from build123d import *

# Parameters (mm, degrees)
FILLET_1_R = 1


with BuildPart() as part:
    # Эскиз2 → Повернуть1 (revolve)
    with BuildSketch(Plane(origin=(0, 0, 0), x_dir=(0, 0, -1), z_dir=(1, 0, 0)), mode=Mode.PRIVATE) as revolve_1_sk:
        Polygon((0, 0), (3, 0), (3, 6.3), (5, 8.3), (5, 9.8), (4, 9.8), (4, 15), (0, 15), align=None)
    revolve(revolve_1_sk.sketch.rotate(Axis((0, 8.655462185, 0), (0, -1, 0)), 180), axis=Axis((0, 8.655462185, 0), (0, -1, 0)))

    # Скругление1
    fillet_1_edges = [part.edges().sort_by_distance(p)[0] for p in [
        (0, 15, -4),
    ]]
    fillet(fillet_1_edges, radius=FILLET_1_R)


solid = part.part
Could you check a few things on this model? Use its own coordinates, in mm. A direction names the side the tool comes from. Give positions to 0.01 mm unless a question says otherwise; leave off trailing zeros. Write each loop counter-clockwise with the first axis right and the second up, starting at its lowest first coordinate (ties: lowest second). Pieces come first, ordered by that corner, then holes. Notation, with made-up numbers: (7, -34.75) -> (48, -34.75) arc R27 ccw to (48, -17.75) -> close; hole circle Ø5 at (61.5, 62). An arc over 180 degrees is marked (long way). Answer as CSV lines item,"result". Start each with the question number.
(1) Please list where these lines run through material, in increasing order: line 1 (X direction, y = 5.25, z = 0); line 2 (Z direction, x = 3.5, y = 14); line 3 (Y direction, x = -4, z = -1.25).
(2) If we section it at A-A, the plane z = 0: Write out the boundary of the cut face in (x, y).
(3) If we section it at D-D, the plane y = 13.75: Write out the boundary of the cut face in (x, z).
(4) Which directions (+Z, -Z, +X, -X, +Y, -Y) give clear straight access to the entire face, cutting with the end or side of a thin tool? Please do faces 1 (the face through (0, 15, 0)), 2 (the face through (-0.9, 3.19, 2.86)), 3 (the face through (3.905, 11.929, -0.867)).
(5) If we section it at B-B, the plane x = 0: Write out the boundary of the cut face in (y, z).
(6) If we section it at C-C, the plane y = 7.75: Write out the boundary of the cut face in (x, z).
(7) I'm going to push flat-ended pins straight in: pin 1 Ø2 at (y, z) = (13, 0) entering from +X; pin 2 Ø1.5 at (x, y) = (3.5, 5) entering from -Z. Where does each tip first touch, or does it pass through?
Answer list:
1,line 1,"-3 to 3"
1,line 2,"-1.94 to 1.94"
1,line 3,"7.49 to 9.8"
2,outline,"(-5, 8.3) -> (-3, 6.3) -> (-3, 0) -> (3, 0) -> (3, 6.3) -> (5, 8.3) -> (5, 9.8) -> (4, 9.8) -> (4, 14) arc R1 ccw to (3, 15) -> (-3, 15) arc R1 ccw to (-4, 14) -> (-4, 9.8) -> (-5, 9.8) -> close"
3,outline,"circle Ø8 at (0, 0)"
4,face 1,"+Z, -Z, +X, -X, +Y"
4,face 2,"-Y"
4,face 3,"+Y"
5,outline,"(0, -3) -> (6.3, -3) -> (8.3, -5) -> (9.8, -5) -> (9.8, -4) -> (14, -4) arc R1 ccw to (15, -3) -> (15, 3) arc R1 ccw to (14, 4) -> (9.8, 4) -> (9.8, 5) -> (8.3, 5) -> (6.3, 3) -> (0, 3) -> close"
6,outline,"circle Ø8.9 at (0, 0)"
7,pin 1,"x = 4"
7,pin 2,"z = -1.2"
